from build123d import *

# Parameters (mm, degrees)
SKETCH2_W            = 111.125
SKETCH2_H            = 193.04
BOSS_EXTRUDE1_DEPTH  = 1.5875
M4_CLEARANCE_HOLE1_D = 4.5
FILLET1_R            = 15.875
SKETCH6_R            = 2.4003
SKETCH6_R_2          = 3
SKETCH6_R_3          = 6.477
SKETCH6_R_4          = 10.762
CUT_EXTRUDE1_DEPTH   = 212.192646736
SKETCH7_W            = 13.97
SKETCH7_H            = 193.04
BOSS_EXTRUDE2_DEPTH  = 1.5875
SKETCH8_W            = 75.32443897
SKETCH8_H            = 38.1
SKETCH8_R            = 10.762
SKETCH8_R_2          = 3
SKETCH8_H_2          = 31.75
SKETCH8_H_3          = 34.487219484
SKETCH8_R_3          = 2.4003
SKETCH8_R_4          = 6.477
SKETCH8_R_5          = 8.9535
CUT_EXTRUDE2_DEPTH   = 1.5875
FILLET2_R            = 9.525
FILLET3_R            = 6.35
FILLET4_R            = 9.525


with BuildPart() as part:
    # Sketch2 → Boss-Extrude1 (new body)
    # profile 1 of 2: a face of its own
    with BuildSketch(Plane.XY.offset(-401.504104662)):
        with Locations((-6.650833159, 105.295051609)):
            Rectangle(SKETCH2_W, SKETCH2_H)
        with BuildLine():
            ThreePointArc((40.429624387, 185.872334563), (40.429624387, 193.650509156), (32.651449794, 193.650509156))
            Line((32.651449794, 193.650509156), (29.670992248, 190.670051609))
            Line((29.670992248, 190.670051609), (-1.150833159, 190.670051609))
            Line((-1.150833159, 190.670051609), (-1.150833159, 194.079751609))
            ThreePointArc((-1.150833159, 194.079751609), (-6.650833159, 199.579751609), (-12.150833159, 194.079751609))
            Line((-12.150833159, 194.079751609), (-12.150833159, 190.670051609))
            Line((-12.150833159, 190.670051609), (-42.972658566, 190.670051609))
            Line((-42.972658566, 190.670051609), (-45.953116112, 193.650509156))
            ThreePointArc((-45.953116112, 193.650509156), (-53.731290705, 193.650509156), (-53.731290705, 185.872334563))
            Line((-53.731290705, 185.872334563), (-50.750833159, 182.891877016))
            Line((-50.750833159, 182.891877016), (-50.750833159, 138.989051609))
            Line((-50.750833159, 138.989051609), (-54.160533159, 138.989051609))
            ThreePointArc((-54.160533159, 138.989051609), (-59.660533159, 133.489051609), (-54.160533159, 127.989051609))
            Line((-54.160533159, 127.989051609), (-50.750833159, 127.989051609))
            Line((-50.750833159, 127.989051609), (-50.750833159, 82.601051609))
            Line((-50.750833159, 82.601051609), (-54.160533159, 82.601051609))
            ThreePointArc((-54.160533159, 82.601051609), (-59.660533159, 77.101051609), (-54.160533159, 71.601051609))
            Line((-54.160533159, 71.601051609), (-50.750833159, 71.601051609))
            Line((-50.750833159, 71.601051609), (-50.750833159, 27.698226203))
            Line((-50.750833159, 27.698226203), (-53.731290705, 24.717768656))
            ThreePointArc((-53.731290705, 24.717768656), (-53.731290705, 16.939594063), (-45.953116112, 16.939594063))
            Line((-45.953116112, 16.939594063), (-42.972658566, 19.920051609))
            Line((-42.972658566, 19.920051609), (-12.150833159, 19.920051609))
            Line((-12.150833159, 19.920051609), (-12.150833159, 16.510351609))
            ThreePointArc((-12.150833159, 16.510351609), (-6.650833159, 11.010351609), (-1.150833159, 16.510351609))
            Line((-1.150833159, 16.510351609), (-1.150833159, 19.920051609))
            Line((-1.150833159, 19.920051609), (29.670992248, 19.920051609))
            Line((29.670992248, 19.920051609), (32.651449794, 16.939594063))
            ThreePointArc((32.651449794, 16.939594063), (40.429624387, 16.939594063), (40.429624387, 24.717768656))
            Line((40.429624387, 24.717768656), (37.449166841, 27.698226203))
            Line((37.449166841, 27.698226203), (37.449166841, 71.601051609))
            Line((37.449166841, 71.601051609), (40.858866841, 71.601051609))
            ThreePointArc((40.858866841, 71.601051609), (46.358866841, 77.101051609), (40.858866841, 82.601051609))
            Line((40.858866841, 82.601051609), (37.449166841, 82.601051609))
            Line((37.449166841, 82.601051609), (37.449166841, 127.989051609))
            Line((37.449166841, 127.989051609), (40.858866841, 127.989051609))
            ThreePointArc((40.858866841, 127.989051609), (46.358866841, 133.489051609), (40.858866841, 138.989051609))
            Line((40.858866841, 138.989051609), (37.449166841, 138.989051609))
            Line((37.449166841, 138.989051609), (37.449166841, 182.891877016))
            Line((37.449166841, 182.891877016), (40.429624387, 185.872334563))
        make_face(mode=Mode.SUBTRACT)
    # profile 2 of 2: a face of its own
    with BuildSketch(Plane.XY.offset(-401.504104662)):
        with BuildLine():
            Line((37.449166841, 182.891877016), (40.429624387, 185.872334563))
            ThreePointArc((40.429624387, 185.872334563), (40.429624387, 193.650509156), (32.651449794, 193.650509156))
            Line((32.651449794, 193.650509156), (29.670992248, 190.670051609))
            Line((29.670992248, 190.670051609), (-1.150833159, 190.670051609))
            Line((-1.150833159, 190.670051609), (-1.150833159, 194.079751609))
            ThreePointArc((-1.150833159, 194.079751609), (-6.650833159, 199.579751609), (-12.150833159, 194.079751609))
            Line((-12.150833159, 194.079751609), (-12.150833159, 190.670051609))
            Line((-12.150833159, 190.670051609), (-42.972658566, 190.670051609))
            Line((-42.972658566, 190.670051609), (-45.953116112, 193.650509156))
            ThreePointArc((-45.953116112, 193.650509156), (-53.731290705, 193.650509156), (-53.731290705, 185.872334563))
            Line((-53.731290705, 185.872334563), (-50.750833159, 182.891877016))
            Line((-50.750833159, 182.891877016), (-50.750833159, 138.989051609))
            Line((-50.750833159, 138.989051609), (-54.160533159, 138.989051609))
            ThreePointArc((-54.160533159, 138.989051609), (-59.660533159, 133.489051609), (-54.160533159, 127.989051609))
            Line((-54.160533159, 127.989051609), (-50.750833159, 127.989051609))
            Line((-50.750833159, 127.989051609), (-50.750833159, 82.601051609))
            Line((-50.750833159, 82.601051609), (-54.160533159, 82.601051609))
            ThreePointArc((-54.160533159, 82.601051609), (-59.660533159, 77.101051609), (-54.160533159, 71.601051609))
            Line((-54.160533159, 71.601051609), (-50.750833159, 71.601051609))
            Line((-50.750833159, 71.601051609), (-50.750833159, 27.698226203))
            Line((-50.750833159, 27.698226203), (-53.731290705, 24.717768656))
            ThreePointArc((-53.731290705, 24.717768656), (-53.731290705, 16.939594063), (-45.953116112, 16.939594063))
            Line((-45.953116112, 16.939594063), (-42.972658566, 19.920051609))
            Line((-42.972658566, 19.920051609), (-12.150833159, 19.920051609))
            Line((-12.150833159, 19.920051609), (-12.150833159, 16.510351609))
            ThreePointArc((-12.150833159, 16.510351609), (-6.650833159, 11.010351609), (-1.150833159, 16.510351609))
            Line((-1.150833159, 16.510351609), (-1.150833159, 19.920051609))
            Line((-1.150833159, 19.920051609), (29.670992248, 19.920051609))
            Line((29.670992248, 19.920051609), (32.651449794, 16.939594063))
            ThreePointArc((32.651449794, 16.939594063), (40.429624387, 16.939594063), (40.429624387, 24.717768656))
            Line((40.429624387, 24.717768656), (37.449166841, 27.698226203))
            Line((37.449166841, 27.698226203), (37.449166841, 71.601051609))
            Line((37.449166841, 71.601051609), (40.858866841, 71.601051609))
            ThreePointArc((40.858866841, 71.601051609), (46.358866841, 77.101051609), (40.858866841, 82.601051609))
            Line((40.858866841, 82.601051609), (37.449166841, 82.601051609))
            Line((37.449166841, 82.601051609), (37.449166841, 127.989051609))
            Line((37.449166841, 127.989051609), (40.858866841, 127.989051609))
            ThreePointArc((40.858866841, 127.989051609), (46.358866841, 133.489051609), (40.858866841, 138.989051609))
            Line((40.858866841, 138.989051609), (37.449166841, 138.989051609))
            Line((37.449166841, 138.989051609), (37.449166841, 182.891877016))
        make_face()
    extrude(amount=BOSS_EXTRUDE1_DEPTH)

    # M4 Clearance Hole1 (through all)
    with Locations(Plane.XY.offset(-399.916604662)):
        with Locations((36.540537091, 189.761421859), (-6.650833159, 194.079751609), (-49.842203409, 189.761421859), (-54.160533159, 133.489051609), (-54.160533159, 77.101051609), (-49.842203409, 20.82868136), (-6.650833159, 16.510351609), (36.540537091, 20.82868136), (40.858866841, 77.101051609), (40.858866841, 133.489051609), (14.260079544, 195.670051609), (-55.750833159, 105.295051609), (-27.561745863, 14.920051609)):
            Hole(M4_CLEARANCE_HOLE1_D / 2)

    # Fillet1
    fillet1_edges = [part.edges().sort_by_distance(p)[0] for p in [
        (-62.213333159, 201.815051609, -400.710354662),
        (-62.213333159, 8.775051609, -400.710354662),
    ]]
    fillet(fillet1_edges, radius=FILLET1_R)

    # Sketch6 → Cut-Extrude1 (cut, through all)
    with BuildSketch(Plane.XY.offset(-399.916604662)):
        with Locations((-34.590833159, 43.382551609)):
            Circle(SKETCH6_R)
        with Locations((21.289166841, 43.382551609)):
            Circle(SKETCH6_R)
        with Locations((-20.884724927, 142.590766631)):
            Circle(SKETCH6_R_2)
        with Locations((7.583058609, 166.225175879)):
            Circle(SKETCH6_R_2)
        with Locations((3.509166841, 43.382551609)):
            Circle(SKETCH6_R_3)
        with Locations((-16.810833159, 43.382551609)):
            Circle(SKETCH6_R_3)
        with Locations((-33.320833159, 123.670051609)):
            Circle(SKETCH6_R_3)
        with Locations((-6.650833159, 154.407971255)):
            Circle(SKETCH6_R_4)
        with Locations((-6.650833159, 94.607131964)):
            Circle(SKETCH6_R_4)
    extrude(amount=-CUT_EXTRUDE1_DEPTH, mode=Mode.SUBTRACT)

    # Sketch7 → Boss-Extrude2 (add)
    with BuildSketch(Plane.XY.offset(-399.916604662)):
        with Locations((55.896666841, 105.295051609)):
            Rectangle(SKETCH7_W, SKETCH7_H)
    extrude(amount=-BOSS_EXTRUDE2_DEPTH)

    # Sketch8 → Cut-Extrude2 (cut)
    # profile 1 of 4: a face of its own
    with BuildSketch(Plane.XY.offset(-399.916604662)):
        with Locations((-6.650833159, 154.407971255)):
            Rectangle(SKETCH8_W, SKETCH8_H)
        with Locations((-6.650833159, 154.407971255)):
            Circle(SKETCH8_R, mode=Mode.SUBTRACT)
        with Locations((7.583058609, 166.225175879)):
            Circle(SKETCH8_R_2, mode=Mode.SUBTRACT)
        with Locations((-20.884724927, 142.590766631)):
            Circle(SKETCH8_R_2, mode=Mode.SUBTRACT)
    # profile 2 of 4: a face of its own
    with BuildSketch(Plane.XY.offset(-399.916604662)):
        with Locations((-6.650833159, 94.607131964)):
            Rectangle(SKETCH8_W, SKETCH8_H_2)
        with Locations((-6.650833159, 94.607131964)):
            Circle(SKETCH8_R, mode=Mode.SUBTRACT)
    # profile 3 of 4: a face of its own
    with BuildSketch(Plane.XY.offset(-399.916604662)):
        with Locations((-6.650833159, 43.601441867)):
            Rectangle(SKETCH8_W, SKETCH8_H_3)
        with Locations((-34.590833159, 43.382551609)):
            Circle(SKETCH8_R_3, mode=Mode.SUBTRACT)
        with Locations((-16.810833159, 43.382551609)):
            Circle(SKETCH8_R_4, mode=Mode.SUBTRACT)
        with Locations((3.509166841, 43.382551609)):
            Circle(SKETCH8_R_4, mode=Mode.SUBTRACT)
        with Locations((21.289166841, 43.382551609)):
            Circle(SKETCH8_R_3, mode=Mode.SUBTRACT)
    # profile 4 of 4: a face of its own
    with BuildSketch(Plane.XY.offset(-399.916604662)):
        with Locations((-33.320833159, 123.670051609)):
            Circle(SKETCH8_R_5)
        with Locations((-33.320833159, 123.670051609)):
            Circle(SKETCH8_R_4, mode=Mode.SUBTRACT)
    extrude(amount=-CUT_EXTRUDE2_DEPTH, mode=Mode.SUBTRACT)

    # Fillet2
    fillet2_edges = [part.edges().sort_by_distance(p)[0] for p in [
        (31.011386326, 135.357971255, -400.710354662),
        (-44.313052644, 135.357971255, -400.710354662),
        (-44.313052644, 173.457971255, -400.710354662),
        (31.011386326, 173.457971255, -400.710354662),
    ]]
    fillet(fillet2_edges, radius=FILLET2_R)

    # Fillet3
    fillet3_edges = [part.edges().sort_by_distance(p)[0] for p in [
        (-44.313052644, 60.845051609, -400.710354662),
        (31.011386326, 60.845051609, -400.710354662),
        (31.011386326, 26.357832125, -400.710354662),
        (-44.313052644, 26.357832125, -400.710354662),
    ]]
    fillet(fillet3_edges, radius=FILLET3_R)

    # Fillet4
    fillet4_edges = [part.edges().sort_by_distance(p)[0] for p in [
        (31.011386326, 110.482131964, -400.710354662),
        (31.011386326, 78.732131964, -400.710354662),
        (-44.313052644, 78.732131964, -400.710354662),
        (-44.313052644, 110.482131964, -400.710354662),
    ]]
    fillet(fillet4_edges, radius=FILLET4_R)


solid = part.part
Part model, mm, in its own coordinate system. Give positions to 0.01 mm unless a question says otherwise; leave off trailing zeros. Write each loop counter-clockwise with the first axis right and the second up, starting at its lowest first coordinate (ties: lowest second). Pieces come first, ordered by that corner, then holes.
1) Pin check, flat tip, straight feed: pin 1 (3.5 mm diameter, centred on x = -54.16, y = 133.49, fed in from -Z). Stop position of the tip, or through.
Resolved:
pin 1: passes through
2) Two-plate mould, pull along X, no slides. Class faces 1 (the face through (37.028, 18.632, -400.721)), 2 (the face through (-57.69, 197.04, -400.7)), 3 (the face through (-1, 128, -401.504)): released by +X, released by -X, zero draft, split by the parting line, or undercut.
Resolved:
face 1: undercut
face 2: released by -X
face 3: zero draft
3) Probe L1, parallel to Y at x = 40.5, z = -400.7; L2, parallel to Y at x = -11.5, z = -400.55; L3, parallel to X at y = 164.5, z = -400.6. List the from-to ranges inside material, lowest first.
Resolved:
L1: y = 8.78 to 74.88, 79.32 to 131.27, 135.71 to 201.82
L2: y = 8.78 to 26.36, 60.85 to 78.73, 110.48 to 135.36, 173.46 to 201.82
L3: x = -62.21 to -44.3, 30.99 to 62.88
4) Cut at B-B on y = 126.5. Write the cut outline in (x, z), then the cut area to 3 significant figures.
Resolved:
outline: (-62.21, -401.5) - (-41.82, -401.5) - (-41.82, -399.92) - (-62.21, -399.92) - close; (-24.83, -401.5) - (62.88, -401.5) - (62.88, -399.92) - (-24.83, -399.92) - close
area: 172 mm2
5) Cut at C-C on z = -400.55. State how many separate pieces and enclosed holes the cut face has, then the cut area to 3 significant figures.
Resolved:
separate pieces: 1
enclosed holes: 17
area: 15,900 mm2
6) Cut at A-A on y = 154.5. Write the cut outline in (x, z), then the cut area to 3 significant figures.
Resolved:
outline: (-62.21, -401.5) - (-44.31, -401.5) - (-44.31, -399.92) - (-62.21, -399.92) - close; (31.01, -401.5) - (62.88, -401.5) - (62.88, -399.92) - (31.01, -399.92) - close
area: 79.0 mm2
